The figure shows three views and two pictorial views of one solid part (mm, origin at its lowest corner). Answer the questions. Round coordinates to 2 decimals unless told otherwise and drop trailing zeros. Order: outer loops, then holes, each group sorted by start corner. A loop starts at its lowest first (then second) coordinate and runs counter-clockwise, first axis right, second up. Notation, with made-up numbers: (79.25, -39.5) -> (103.25, -39.5) arc R18 ccw to (103.25, -15.5) -> close; hole circle Ø4 at (63, 46.25). An arc over 180 degrees is marked (long way). Answer in a Markdown table with one row per item. Add a question column.
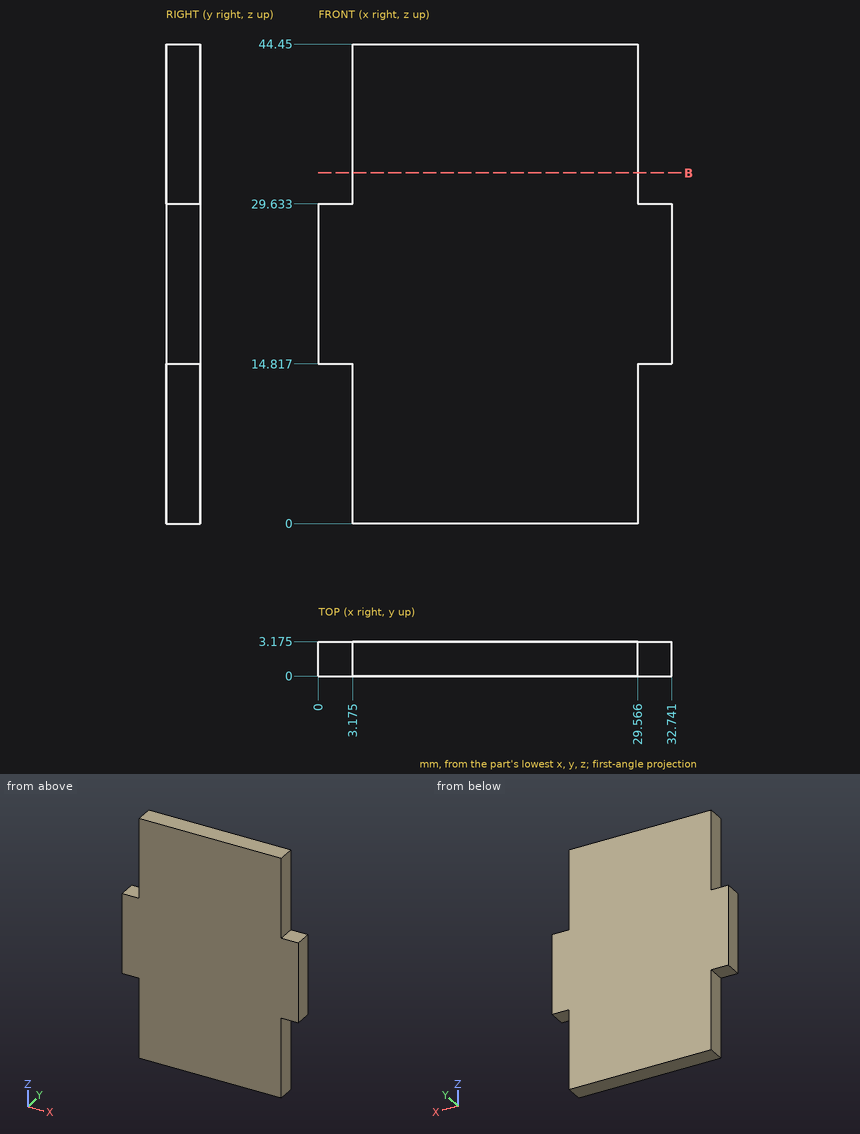
1. The part is cut by section B-B (z = 32.5). Give the vertices of the cut face in (x, y) (1 decimal).
2. Each of these flat-tipped pins is pushed along its axis until it touches: pin 1 (1.6 mm diameter, centred on y = 2, z = 33.5, fed in from -X) (3 decimals); pin 2 (1 mm diameter, centred on x = 31, y = 1, fed in from +Z); pin 3 (1.6 mm diameter, centred on y = 1.5, z = 34, fed in from +X). Where does it stop, or does it pass through?
3. Straight lines are drawn through the part: line 1 along X through (y, z) = (0.25, 9.5) (1 decimal); line 2 along Z through (x, y) = (2, 1.55). For each, find the intervals that lie inside material, in ascending order.
Report:
| question | item | result |
|---|---|---|
| 1 | outline | (3.2, 0) -> (29.6, 0) -> (29.6, 3.2) -> (3.2, 3.2) -> close |
| 2 | pin 1 | stops at x = 3.175 |
| 2 | pin 2 | stops at z = 29.63 |
| 2 | pin 3 | stops at x = 29.57 |
| 3 | line 1 | x = 3.2 to 29.6 |
| 3 | line 2 | z = 14.82 to 29.63 |
